from build123d import *

# Parameters (mm, degrees)
SKETCH_1_R          = 3
EXTRUDE_1_DEPTH     = 20
SKETCH_2_R          = 7
CUT_EXTRUDE_1_DEPTH = 4


with BuildPart() as part:
    # 스케치1 → 보스-돌출1 (new body, symmetric)
    with BuildSketch(Plane.XY):
        with BuildLine():
            Line((0, 7), (0, 44))
            ThreePointArc((0, 44), (0.878679656, 46.121320344), (3, 47))
            Line((3, 47), (7.5, 47))
            ThreePointArc((7.5, 47), (15.226747122, 41.07301204), (11.504409953, 32.074344729))
            Line((11.504409953, 32.074344729), (19, 16))
            Line((19, 16), (44.136675312, 9.26464815))
            ThreePointArc((44.136675312, 9.26464815), (45.397872906, 9.201846853), (46.573187235, 9.663582275))
            ThreePointArc((46.573187235, 9.663582275), (54.780575213, 10.050336947), (59, 3))
            ThreePointArc((59, 3), (58.121320344, 0.878679656), (56, 0))
            Line((56, 0), (7, 0))
            ThreePointArc((7, 0), (2.050252532, 2.050252532), (0, 7))
        make_face()
        with Locations((7, 7)):
            Circle(SKETCH_1_R, mode=Mode.SUBTRACT)
    extrude(amount=EXTRUDE_1_DEPTH, both=True)

    # 스케치2 → 컷-돌출1 (cut)
    with BuildSketch(Plane.XZ):
        with Locations((49, 0)):
            Circle(SKETCH_2_R)
    extrude(amount=-CUT_EXTRUDE_1_DEPTH, mode=Mode.SUBTRACT)


solid = part.part
Can you work these out from the model? Positions are in its coordinate system, mm. A direction names the side the tool comes from. Give positions to 0.01 mm unless a question says otherwise; leave off trailing zeros. Order: outer loops, then holes, each group sorted by start corner. A loop starts at its lowest first (then second) coordinate and runs counter-clockwise, first axis right, second up. Notation, with made-up numbers: M 67.25,88 L 80.25,88 A9 ccw 80.25,104 Z; hole C -1.75,89 d4. An arc over 180 degrees is marked long. Use a Markdown table: item, result. Add a question column.
Item 1: We'd pull the mould along X, two halves only. Please class faces 4 (the cylindrical face through (0.86, 46.1, 0.28)), 5 (the flat face through (5, 47, 0)), 6 (the cylindrical face through (45.38, 9.2, 0.28)): +X half, -X half, draft (parallel to the pull), parting line (faces both ways), or undercut.
Item 2: Will these pins go through, and if not, where does the flat tip stop? pin 1 (11 mm diameter, centred on x = 49, z = 0, fed in from +Y); pin 2 (4 mm diameter, centred on x = 51.5, z = -3, fed in from -Y); pin 3 (4 mm diameter, centred on x = 46.5, z = 8, fed in from +Y).
Item 3: Suppose I cut it at A-A (x = 13). List the corners of the cut face in (y, z) for me, then the cut area to 3 significant figures.
Item 4: Suppose I cut it at C-C (x = 49). List the corners of the cut face in (y, z) for me.
Item 5: If I drill on L1, parallel to Y at x = 7, z = -5; L2, parallel to Z at x = 49, y = 2.1; L3, parallel to X at y = 5, z = -2, over which ranges is the centre line in solid material (lowest first)? Write a range as [from, to].
Item 6: Suppose I cut it at B-B (z = 11). List the corners of the cut face in (x, y) for me.
Item 7: Suppose I cut it at D-D (y = 20). List the corners of the cut face in (x, z) for me.
Item 8: For faces 1 (the flat face through (15.2, 24.15, 0.28)), 2 (the flat face through (31.39, 12.68, 0.28)), 3 (the cylindrical face through (55.677, 1.972, 2.103)), which set-ups out of +Z, -Z, +X, -X, +Y, -Y let a thin tool reach every point of the face, with its end or its side?
Answer sheet:
| question | item | result |
|---|---|---|
| 1 | face 4 | -X half |
| 1 | face 5 | draft |
| 1 | face 6 | undercut |
| 2 | pin 1 | stops at y = 11 |
| 2 | pin 2 | stops at y = 4 |
| 2 | pin 3 | stops at y = 10.6 |
| 3 | outline | M 0,-20 L 28.87,-20 L 28.87,20 L 0,20 Z; M 33.19,-20 L 44.81,-20 L 44.81,20 L 33.19,20 Z |
| 3 | area | 1,620 mm² |
| 4 | outline | M 0,-20 L 10.75,-20 L 10.75,20 L 0,20 L 0,7 L 4,7 L 4,-7 L 0,-7 Z |
| 5 | L1 | y = [0, 4], [10, 47] |
| 5 | L2 | z = [-20, -7], [7, 20] |
| 5 | L3 | x = [0.29, 4.76], [9.24, 58.75] |
| 6 | outline | M 0,7 A7 ccw 7,0 L 56,0 A3 ccw 59,3 A8 ccw 46.57,9.66 A3 cw 44.14,9.26 L 19,16 L 11.5,32.07 A8 ccw 7.5,47 L 3,47 A3 ccw 0,44 Z; hole C 7,7 d6 |
| 7 | outline | M 0,-20 L 17.13,-20 L 17.13,20 L 0,20 Z |
| 8 | face 1 | +Z, -Z, +X |
| 8 | face 2 | +Z, -Z, +Y |
| 8 | face 3 | -Y |
